Work out the finished part from the listing and answer in its coordinate system (mm). A direction names the side the tool comes from. Round coordinates to 2 decimals unless told otherwise and drop trailing zeros. Loops run counter-clockwise (first coordinate to the right, second up) from the corner with the lowest first, then second, coordinate; pieces in that order, holes last. Notation, with made-up numbers: (71, 69) - (79, 69) arc R19 cw to (79, 105) - close; hole circle Ø8 at (28, 64.5). An arc over 180 degrees is marked (long way). Answer as CSV lines item,"result". Start each with the question number.
Q1. The mould has two halves that part along Y. Classify faces 5 (the face through (-29, 89, 59)), 6 (the face through (-58.57, 57.2, 57.01)): +Y half, -Y half, draft (parallel to the pull), parting line (faces both ways), or undercut.
Q2. Section A-A on x = 65 is taken. Write down the section's boundary in (y, z).
Q3. Section D-D on y = 64 is taken. Write down the section's boundary in (x, z), then the cut area to 3 significant figures.
Q4. Each of these flat-tipped pins is pushed along its axis until it touches: pin 1 Ø3.5 at (x, z) = (-67, 58) entering from -Y; pin 2 Ø7.5 at (x, z) = (-27.5, 51) entering from -Y; pin 3 Ø3.5 at (x, y) = (-69, 41.75) entering from -Z; pin 4 Ø3.5 at (x, y) = (-67, 31.5) entering from -Z. Where does it stop, or does it pass through?
Q5. Section C-C on x = -69 is taken. Write down the section's boundary in (y, z).
Q6. For faces 1 (the face through (-54.5, 50, 58)), 2 (the face through (2.2, 3.9, 59)), 3 (the face through (-67, 90, 57)), 4 (the face through (-30, 55.5, 49)), determine the directions among +Z, -Z, +X, -X, +Y, -Y from which every point of the face is accessible in a straight line to the end or side of a thin tool.
Q7. Section B-B on z = 45.5 is taken. Count the separate pieces of the cut face and the enclosed holes in it, then the cut area to 3 significant figures.
Q8. Straight lines are drawn through the part: L1, parallel to Y at x = 65, z = 57; L2, parallel to X at y = 91.5, z = 57.25; L3, parallel to X at y = 58.5, z = 56.75. For each, find the intervals that lie inside material, in ascending order. Write a range as [from, to].
```python
from build123d import *

# Parameters (mm, degrees)
SKETCH1_W                 = 150
SKETCH1_H                 = 4
BOSS_EXTRUDE1_DEPTH       = 100
SKETCH9_W                 = 4
SKETCH9_H                 = 100
BOSS_EXTRUDE4_DEPTH       = 5.8
SKETCH10_W                = 20
SKETCH10_H                = 1.5
BOSS_EXTRUDE5_DEPTH       = 15
LPATTERN1_COUNT           = 2
LPATTERN1_PITCH           = 60
LPATTERN2_COUNT           = 2
LPATTERN2_PITCH           = 25
LPATTERN2_COPY_1_SKETCH_W = 20
LPATTERN2_COPY_1_SKETCH_H = 1.5
LPATTERN2_COPY_1_DEPTH    = 15
LPATTERN3_COUNT           = 2
LPATTERN3_PITCH           = 4
LPATTERN3_COPY_1_SKETCH_W = 20
LPATTERN3_COPY_1_SKETCH_H = 1.5
LPATTERN3_COPY_1_DEPTH    = 15
LPATTERN3_COPY_2_SKETCH_W = 20
LPATTERN3_COPY_2_SKETCH_H = 1.5
LPATTERN3_COPY_2_DEPTH    = 15
LPATTERN3_COPY_3_SKETCH_W = 20
LPATTERN3_COPY_3_SKETCH_H = 1.5
LPATTERN3_COPY_3_DEPTH    = 15
SKETCH12_R                = 3.5
CUT_EXTRUDE2_DEPTH        = 2
CUT_EXTRUDE3_REACH        = 216.198
SKETCH14_R                = 2.25
LPATTERN4_COUNT           = 3
LPATTERN4_PITCH           = 60
SKETCH16_R                = 3
CUT_EXTRUDE4_DEPTH        = 2
CUT_EXTRUDE5_REACH        = 125.072
SKETCH18_R                = 1.5
LPATTERN5_COUNT           = 2
LPATTERN5_PITCH           = 25
SKETCH19_W                = 10
SKETCH19_H                = 7
CUT_EXTRUDE6_DEPTH        = 3
LPATTERN6_COUNT           = 2
LPATTERN6_PITCH           = 55
CUT_EXTRUDE7_REACH        = 127.897
SKETCH20_W                = 11
SKETCH20_H                = 78
FILLET4_R                 = 2
LPATTERN7_COUNT           = 3
LPATTERN7_PITCH           = 50
FILLET4_OF_LPATTERN7_R    = 2
SKETCH21_W                = 8
SKETCH21_H                = 10
CUT_EXTRUDE8_DEPTH        = 3
LPATTERN8_COUNT           = 2
LPATTERN8_PITCH           = 60
SKETCH23_R                = 3
CUT_EXTRUDE9_DEPTH        = 2
CUT_EXTRUDE10_REACH       = 106.668
SKETCH25_R                = 1.5
SKETCH27_R                = 3
CUT_EXTRUDE11_DEPTH       = 2
CUT_EXTRUDE12_REACH       = 131.476
SKETCH29_R                = 1.5
LPATTERN10_COUNT          = 2
LPATTERN10_PITCH          = 125


with BuildPart() as part:
    # Sketch1 → Boss-Extrude1 (new body)
    with BuildSketch(Plane(origin=(0, 0, 0), x_dir=(1, 0, 0), z_dir=(0, 1, 0))):
        with Locations((0, -58)):
            Rectangle(SKETCH1_W, SKETCH1_H)
    extrude(amount=BOSS_EXTRUDE1_DEPTH)

    # Sketch9 → Boss-Extrude4 (add)
    with BuildSketch(Plane(origin=(0, 0, 56), x_dir=(-1, 0, 0), z_dir=(0, 0, -1))):
        with Locations((-73, 50)):
            Rectangle(SKETCH9_W, SKETCH9_H)
    extrude(amount=BOSS_EXTRUDE4_DEPTH)

    # Sketch10 → Boss-Extrude5 (add)
    with BuildSketch(Plane(origin=(0, 0, 56), x_dir=(-1, 0, 0), z_dir=(0, 0, -1))):
        with Locations((-30, 50.75)):
            Rectangle(SKETCH10_W, SKETCH10_H)
    boss_extrude5 = extrude(amount=BOSS_EXTRUDE5_DEPTH)

    # LPattern1: Boss-Extrude5 ×2
    with Locations(*[(-i * LPATTERN1_PITCH, 0, 0) for i in range(1, LPATTERN1_COUNT)]):
        add(boss_extrude5)

    # LPattern2: Boss-Extrude5 ×2
    with Locations(*[(0, i * LPATTERN2_PITCH, 0) for i in range(1, LPATTERN2_COUNT)]):
        add(boss_extrude5)

    # LPattern2 copy 1 sketch → LPattern2 copy 1 (add)
    with BuildSketch(Plane(origin=(-60, 25, 56), x_dir=(-1, 0, 0), z_dir=(0, 0, -1))):
        with Locations((-30, 50.75)):
            Rectangle(LPATTERN2_COPY_1_SKETCH_W, LPATTERN2_COPY_1_SKETCH_H)
    extrude(amount=LPATTERN2_COPY_1_DEPTH)

    # LPattern3: Boss-Extrude5 ×2
    with Locations(*[(0, i * LPATTERN3_PITCH, 0) for i in range(1, LPATTERN3_COUNT)]):
        add(boss_extrude5)

    # LPattern3 copy 1 sketch → LPattern3 copy 1 (add)
    with BuildSketch(Plane(origin=(-60, 4, 56), x_dir=(-1, 0, 0), z_dir=(0, 0, -1))):
        with Locations((-30, 50.75)):
            Rectangle(LPATTERN3_COPY_1_SKETCH_W, LPATTERN3_COPY_1_SKETCH_H)
    extrude(amount=LPATTERN3_COPY_1_DEPTH)

    # LPattern3 copy 2 sketch → LPattern3 copy 2 (add)
    with BuildSketch(Plane(origin=(0, 29, 56), x_dir=(-1, 0, 0), z_dir=(0, 0, -1))):
        with Locations((-30, 50.75)):
            Rectangle(LPATTERN3_COPY_2_SKETCH_W, LPATTERN3_COPY_2_SKETCH_H)
    extrude(amount=LPATTERN3_COPY_2_DEPTH)

    # LPattern3 copy 3 sketch → LPattern3 copy 3 (add)
    with BuildSketch(Plane(origin=(-60, 29, 56), x_dir=(-1, 0, 0), z_dir=(0, 0, -1))):
        with Locations((-30, 50.75)):
            Rectangle(LPATTERN3_COPY_3_SKETCH_W, LPATTERN3_COPY_3_SKETCH_H)
    extrude(amount=LPATTERN3_COPY_3_DEPTH)

    # Sketch12 → Cut-Extrude2 (cut)
    with BuildSketch(Plane(origin=(118.42090966, 9.556382744, 60), x_dir=(1, 0, 0), z_dir=(0, 0, 1))):
        with Locations((-53.42090966, -3.556382744)):
            Circle(SKETCH12_R)
    cut_extrude2 = extrude(amount=-CUT_EXTRUDE2_DEPTH, mode=Mode.SUBTRACT)

    # Sketch14 → Cut-Extrude3 (cut, up to next)
    with BuildSketch(Plane(origin=(118.42090966, 9.556382744, 58), x_dir=(1, 0, 0), z_dir=(0, 0, 1)), mode=Mode.PRIVATE) as cut_extrude3_sk1:
        with Locations((-53.42090966, -3.556382744)):
            Circle(SKETCH14_R)
    cut_extrude3_tool1 = extrude(cut_extrude3_sk1.sketch, amount=-CUT_EXTRUDE3_REACH, mode=Mode.PRIVATE) & part.part
    cut_extrude3 = cut_extrude3_tool1.solids().sort_by_distance((65, 6, 58))[0]
    add(cut_extrude3, mode=Mode.SUBTRACT)

    # LPattern4: Cut-Extrude2, Cut-Extrude3 ×3
    with Locations(*[(-i * LPATTERN4_PITCH, 0, 0) for i in range(1, LPATTERN4_COUNT)]):
        add(cut_extrude2, mode=Mode.SUBTRACT)
        add(cut_extrude3, mode=Mode.SUBTRACT)

    # Sketch16 → Cut-Extrude4 (cut)
    with BuildSketch(Plane(origin=(-5.380870304, 91.632593669, 60), x_dir=(1, 0, 0), z_dir=(0, 0, 1))):
        with Locations((-54.619129696, -9.882593669)):
            Circle(SKETCH16_R)
    cut_extrude4 = extrude(amount=-CUT_EXTRUDE4_DEPTH, mode=Mode.SUBTRACT)

    # Sketch18 → Cut-Extrude5 (cut, up to next)
    with BuildSketch(Plane(origin=(-5.380870304, 91.632593669, 58), x_dir=(1, 0, 0), z_dir=(0, 0, 1)), mode=Mode.PRIVATE) as cut_extrude5_sk1:
        with Locations((-54.619129696, -9.882593669)):
            Circle(SKETCH18_R)
    cut_extrude5_tool1 = extrude(cut_extrude5_sk1.sketch, amount=-CUT_EXTRUDE5_REACH, mode=Mode.PRIVATE) & part.part
    cut_extrude5 = cut_extrude5_tool1.solids().sort_by_distance((-60, 81.75, 58))[0]
    add(cut_extrude5, mode=Mode.SUBTRACT)

    # LPattern5: Cut-Extrude4, Cut-Extrude5 ×2
    with Locations(*[(0, -i * LPATTERN5_PITCH, 0) for i in range(1, LPATTERN5_COUNT)]):
        add(cut_extrude4, mode=Mode.SUBTRACT)
        add(cut_extrude5, mode=Mode.SUBTRACT)

    # Sketch19 → Cut-Extrude6 (cut)
    with BuildSketch(Plane(origin=(0, 0, 56), x_dir=(-1, 0, 0), z_dir=(0, 0, -1))):
        with Locations((67.5, 86.5)):
            Rectangle(SKETCH19_W, SKETCH19_H)
    cut_extrude6 = extrude(amount=-CUT_EXTRUDE6_DEPTH, mode=Mode.SUBTRACT)

    # LPattern6: Cut-Extrude6 ×2
    with Locations(*[(0, -i * LPATTERN6_PITCH, 0) for i in range(1, LPATTERN6_COUNT)]):
        add(cut_extrude6, mode=Mode.SUBTRACT)

    # Sketch20 → Cut-Extrude7 (cut, up to next)
    with BuildSketch(Plane(origin=(0, 0, 56), x_dir=(-1, 0, 0), z_dir=(0, 0, -1)), mode=Mode.PRIVATE) as cut_extrude7_sk1:
        with Locations((49, 51)):
            Rectangle(SKETCH20_W, SKETCH20_H)
    cut_extrude7_tool1 = extrude(cut_extrude7_sk1.sketch, amount=-CUT_EXTRUDE7_REACH, mode=Mode.PRIVATE) & part.part
    cut_extrude7 = cut_extrude7_tool1.solids().sort_by_distance((-49, 51, 56))[0]
    add(cut_extrude7, mode=Mode.SUBTRACT)

    # Fillet4
    fillet4_edges = [part.edges().sort_by_distance(p)[0] for p in [
        (-43.5, 12, 58),
        (-43.5, 90, 58),
        (-54.5, 90, 58),
        (-54.5, 12, 58),
    ]]
    fillet(fillet4_edges, radius=FILLET4_R)

    # LPattern7: Cut-Extrude7 ×3
    with Locations(*[(i * LPATTERN7_PITCH, 0, 0) for i in range(1, LPATTERN7_COUNT)]):
        add(cut_extrude7, mode=Mode.SUBTRACT)

    # Fillet4 of LPattern7
    fillet4_of_lpattern7_edges = [part.edges().sort_by_distance(p)[0] for p in [
        (6.5, 12, 58),
        (6.5, 90, 58),
        (-4.5, 90, 58),
        (-4.5, 12, 58),
        (56.5, 12, 58),
        (56.5, 90, 58),
        (45.5, 90, 58),
        (45.5, 12, 58),
    ]]
    fillet(fillet4_of_lpattern7_edges, radius=FILLET4_OF_LPATTERN7_R)

    # Sketch21 → Cut-Extrude8 (cut)
    with BuildSketch(Plane(origin=(0, 0, 56), x_dir=(-1, 0, 0), z_dir=(0, 0, -1))):
        with Locations((29, 88.538707867)):
            Rectangle(SKETCH21_W, SKETCH21_H)
    cut_extrude8 = extrude(amount=-CUT_EXTRUDE8_DEPTH, mode=Mode.SUBTRACT)

    # LPattern8: Cut-Extrude8 ×2
    with Locations(*[(i * LPATTERN8_PITCH, 0, 0) for i in range(1, LPATTERN8_COUNT)]):
        add(cut_extrude8, mode=Mode.SUBTRACT)

    # Sketch23 → Cut-Extrude9 (cut)
    with BuildSketch(Plane(origin=(-14.094781426, 47.764709476, 60), x_dir=(1, 0, 0), z_dir=(0, 0, 1))):
        with Locations((-54.905218574, -6.014709476)):
            Circle(SKETCH23_R)
    extrude(amount=-CUT_EXTRUDE9_DEPTH, mode=Mode.SUBTRACT)

    # Sketch25 → Cut-Extrude10 (cut, up to next)
    with BuildSketch(Plane(origin=(-14.094781426, 47.764709476, 58), x_dir=(1, 0, 0), z_dir=(0, 0, 1)), mode=Mode.PRIVATE) as cut_extrude10_sk1:
        with Locations((-54.905218574, -6.014709476)):
            Circle(SKETCH25_R)
    cut_extrude10_tool1 = extrude(cut_extrude10_sk1.sketch, amount=-CUT_EXTRUDE10_REACH, mode=Mode.PRIVATE) & part.part
    add(cut_extrude10_tool1.solids().sort_by_distance((-69, 41.75, 58))[0], mode=Mode.SUBTRACT)

    # Sketch27 → Cut-Extrude11 (cut)
    with BuildSketch(Plane(origin=(-5.434124332, 100.026831424, 60), x_dir=(1, 0, 0), z_dir=(0, 0, 1))):
        with Locations((-54.565875668, -5.026831424)):
            Circle(SKETCH27_R)
    cut_extrude11 = extrude(amount=-CUT_EXTRUDE11_DEPTH, mode=Mode.SUBTRACT)

    # Sketch29 → Cut-Extrude12 (cut, up to next)
    with BuildSketch(Plane(origin=(-5.434124332, 100.026831424, 58), x_dir=(1, 0, 0), z_dir=(0, 0, 1)), mode=Mode.PRIVATE) as cut_extrude12_sk1:
        with Locations((-54.565875668, -5.026831424)):
            Circle(SKETCH29_R)
    cut_extrude12_tool1 = extrude(cut_extrude12_sk1.sketch, amount=-CUT_EXTRUDE12_REACH, mode=Mode.PRIVATE) & part.part
    cut_extrude12 = cut_extrude12_tool1.solids().sort_by_distance((-60, 95, 58))[0]
    add(cut_extrude12, mode=Mode.SUBTRACT)

    # LPattern10: Cut-Extrude11, Cut-Extrude12 ×2
    with Locations(*[(i * LPATTERN10_PITCH, 0, 0) for i in range(1, LPATTERN10_COUNT)]):
        add(cut_extrude11, mode=Mode.SUBTRACT)
        add(cut_extrude12, mode=Mode.SUBTRACT)


solid = part.part
```
Findings:
1,face 5,"undercut"
1,face 6,"undercut"
2,outline,"(0, 56) - (3.75, 56) - (3.75, 58) - (2.5, 58) - (2.5, 60) - (0, 60) - close; (8.25, 56) - (93.5, 56) - (93.5, 58) - (92, 58) - (92, 60) - (9.5, 60) - (9.5, 58) - (8.25, 58) - close; (96.5, 56) - (100, 56) - (100, 60) - (98, 60) - (98, 58) - (96.5, 58) - close"
3,outline,"(-75, 56) - (-54.5, 56) - (-54.5, 60) - (-75, 60) - close; (-43.5, 56) - (-4.5, 56) - (-4.5, 60) - (-43.5, 60) - close; (6.5, 56) - (45.5, 56) - (45.5, 60) - (6.5, 60) - close; (56.5, 56) - (71, 56) - (71, 50.2) - (75, 50.2) - (75, 60) - (56.5, 60) - close"
3,area,"491 mm^2"
4,pin 1,"stops at y = 0"
4,pin 2,"stops at y = 50"
4,pin 3,"stops at z = 56"
4,pin 4,"stops at z = 59"
5,outline,"(0, 56) - (28, 56) - (28, 59) - (35, 59) - (35, 56) - (40.25, 56) - (40.25, 58) - (38.75, 58) - (38.75, 60) - (0, 60) - close; (43.25, 56) - (83, 56) - (83, 59) - (90, 59) - (90, 56) - (100, 56) - (100, 60) - (44.75, 60) - (44.75, 58) - (43.25, 58) - close"
6,face 1,"+Z, -Z"
6,face 2,"+Z"
6,face 3,"-Z"
6,face 4,"-Z, -X"
7,separate pieces,"8"
7,enclosed holes,"0"
7,area,"240 mm^2"
8,L1,"y = [0, 3.75], [8.25, 93.5], [96.5, 100]"
8,L2,"x = [-75, -33], [-25, 27], [35, 75]"
8,L3,"x = [-75, -54.5], [-43.5, -4.5], [6.5, 45.5], [56.5, 75]"
